Work out the finished part from the listing and answer in its coordinate system (mm). Face numbers are marked on the shaded views. A direction names the side the tool comes from. Round coordinates to 2 decimals unless told otherwise and drop trailing zeros. Order: outer loops, then holes, each group sorted by start corner. A loop starts at its lowest first (then second) coordinate and runs counter-clockwise, first axis right, second up. Notation, with made-up numbers: (46, 54.5) - (90, 54.5) arc R10 cw to (90, 67.5) - close; hole circle Ø6 at (-29, 31.5). An arc over 180 degrees is marked (long way). Use one line per item in the form item = value. Start each with the question number.
Q1. The part is cut by section C-C on x = 8. Determine the outline of the cut face in (y, z), plus the area to 3 significant figures.
Q2. Find the intervals of material crossed by line 1 (Z direction, x = 8, y = -10); line 2 (Z direction, x = 17.25, y = -10); line 3 (X direction, y = -18, z = -43), in increasing order. Write a range as [from, to].
Q3. Which of the six approach directions +Z, -Z, +X, -X, +Y, -Y give full straight-line access (tool end or side, diameter ignored) to the marked faces 1 and 2?
Q4. For a pull along Y with two mould halves and no side action, classify the marked faces 3, 4 and 5 as +Y half, -Y half, draft (parallel to the pull), parting line (faces both ways), or undercut.
Q5. Given P1, Ø1.2, axis at y = -9.5, z = -11.5, coming from the +X side; P2, Ø1.1, axis at x = 16, z = -21, coming from the +Y side; P3, Ø1.1, axis at x = 16.5, z = -12.5, coming from the -Y side, each flat-ended and moving along its own axis, determine where each tip first touches the part or whether it passes through.
Q6. The part is cut by section A-A on y = -10. State how many separate pieces and enclosed holes the cut face has, plus the area to 3 significant figures.
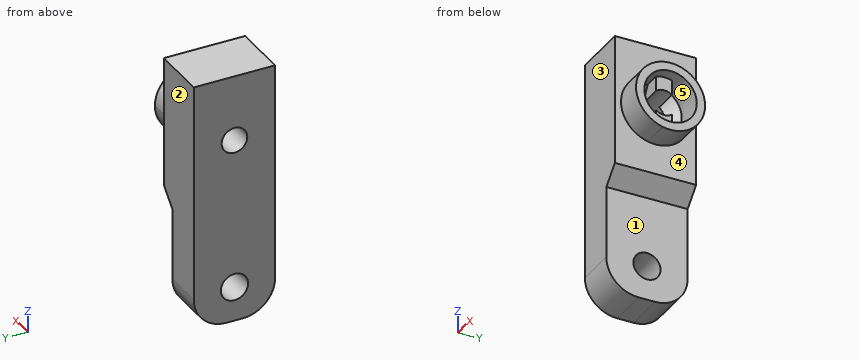
from build123d import *

# Parameters (mm, degrees)
F0_W      = 20
F0_H      = 62
F1_DEPTH  = 14
F2_R      = 8.5
F3_DEPTH  = 7
F5_D      = 12.9
F5_DEPTH  = 7
F5_TIP    = 3.8755509927
F6_W      = 3.8587664786
F6_H      = 16.5562349188
F7_DEPTH  = 11.59683
F9_D      = 6.3
F10_R     = 6.45
F11_DEPTH = 3
F12_R     = 8
F13_R     = 8
F14_W     = 4
F14_H     = 37.0940975845
F15_DEPTH = 25
F17_D     = 6.7
F18_SIZE  = 3.99999


# Not quite as in the source:
# - a fillet or chamfer is up to 0.001 mm smaller than in the source, because OpenCascade refuses the exact size


with BuildPart() as f1:
    # F0 (on Right) → F1 (new body)
    with BuildSketch(Plane.YZ):
        with Locations((-10, -31)):
            Rectangle(F0_W, F0_H)
    extrude(amount=F1_DEPTH)

    # F2 (on face) → F3 (join)
    with BuildSketch(Plane.YZ.offset(14)):
        with Locations((-10, -16.2361655384)):
            Circle(F2_R)
    extrude(amount=F3_DEPTH)

    # F5
    with Locations(Plane.YZ.offset(21)):
        with Locations((-10, -16.2361655384)):
            Hole(F5_D / 2, depth=F5_DEPTH)
            with Locations((0, 0, -(F5_DEPTH + F5_TIP / 2))):  # 118° drill point
                Cone(0, F5_D / 2, F5_TIP, mode=Mode.SUBTRACT)

    # F6 (on face) → F7 (join)
    with BuildSketch(Plane.YZ.offset(21)):
        with Locations((-10.015449224, -16.2397662935)):
            Rectangle(F6_W, F6_H)
    extrude(amount=-F7_DEPTH)

    # F9 (through all)
    with Locations(Plane.YZ.offset(21)):
        with Locations((-10, -16.2361655384)):
            Hole(F9_D / 2)

    # F10 (on face) → F11 (cut)
    with BuildSketch(Plane.YZ.offset(21)):
        with Locations((-10, -16.2361655384)):
            Circle(F10_R)
    extrude(amount=-F11_DEPTH, mode=Mode.SUBTRACT)

    # F12
    f12_edges = [f1.edges().sort_by_distance(p)[0] for p in [
        (7, 0, -62),
    ]]
    fillet(f12_edges, radius=F12_R)

    # F13
    f13_edges = [f1.edges().sort_by_distance(p)[0] for p in [
        (7, -20, -62),
    ]]
    fillet(f13_edges, radius=F13_R)

    # F14 (on face) → F15 (cut)
    with BuildSketch(Plane.XZ.offset(20)):
        with Locations((12, -50.7526341826)):
            Rectangle(F14_W, F14_H)
    extrude(amount=-F15_DEPTH, mode=Mode.SUBTRACT)

    # F17 (through all)
    with Locations(Plane(origin=(0, 0, 0), x_dir=(0, -1, 0), z_dir=(-1, 0, 0))):
        with Locations((10, -53.5)):
            Hole(F17_D / 2)

    # F18 (size 4 in the source; OpenCascade refuses exactly that, so slightly less here)
    f18_edges = [f1.edges().sort_by_distance(p)[0] for p in [
        (10, -10, -32.205585),
    ]]
    chamfer(f18_edges, length=F18_SIZE)


solid = f1.part
Found:
q1.outline = (-20, -54) arc R8 ccw to (-12, -62) - (-8, -62) arc R8 ccw to (0, -54) - (0, 0) - (-20, 0) - close; hole circle Ø6.7 at (-10, -53.5); hole circle Ø6.3 at (-10, -16.24)
q1.area = 1,150 mm²
q2.line_1 = [-62, -56.85], [-50.15, -19.39], [-13.09, 0]
q2.line_2 = [-24.74, -19.39], [-13.09, -7.74]
q2.line_3 = [0, 10]
q3.face_1 = -Z, +X, +Y, -Y
q3.face_2 = +Z, -Z, +X, -X, +Y
q4.face_3 = -Y half
q4.face_4 = draft
q4.face_5 = undercut
q5.P1 = 18
q5.P2 = -2.62
q5.P3 = -17.88
q6.separate_pieces = 3
q6.enclosed_holes = 0
q6.area = 657 mm²
